Answer from the drawing. Dimensions are ordinates in mm from the lowest x, y and z of the part. A direction names the side the tool comes from. Round coordinates to 2 decimals unless told otherwise and drop trailing zeros. Order: outer loops, then holes, each group sorted by start corner. A loop starts at its lowest first (then second) coordinate and runs counter-clockwise, first axis right, second up. Notation, with made-up numbers: M -8,74.5 L -1,74.5 A15 cw -1,96.5 Z; hole C 32,4.25 d11. An arc over 180 degrees is marked long. Write item = value, one per line. Start each with the question number.
(1) A cutting plane is placed at C-C, the plane y = 20.5. Determine the outline of the cut face in (x, z).
(2) Each of these flat-tipped pins is pushed along its axis until it touches: pin 1 (1.5 mm diameter, centred on x = 3.5, y = 13, fed in from +Z); pin 2 (1.5 mm diameter, centred on x = 1.5, y = 11.5, fed in from -Z); pin 3 (2.5 mm diameter, centred on x = 2, z = 4.5, fed in from +Y). Where does it stop, or does it pass through?
(3) Which of the six approach directions +Z, -Z, +X, -X, +Y, -Y give full straight-line access (tool end or side, diameter ignored) to the marked faces 4, 5 and 6?
(4) Straight lines are drawn through the part: probe 1 along Y at (x, z) = (4.5, 0.3); probe 2 along Z at (x, y) = (4.4, 15.5); probe 3 along Z at (x, y) = (0.3, 20.5). For each, find the intervals that lie inside material, in ascending order. Write a range as from..to.
(5) A cutting plane is placed at B-B, the plane x = 1.25. Determine the outline of the cut face in (y, z), and give its area (3 significant figures).
(6) For a pull along Y with two mould halves and no side action, classify the marked faces 1, 2 and 3 as released by +Y, released by -Y, zero draft, split by the parting line, or undercut.
(7) A cutting plane is placed at A-A, the plane z = 0.8. Determine the outline of the cut face in (x, y).
(8) A cutting plane is placed at D-D, the plane z = 4.4. Determine the outline of the cut face in (x, y).
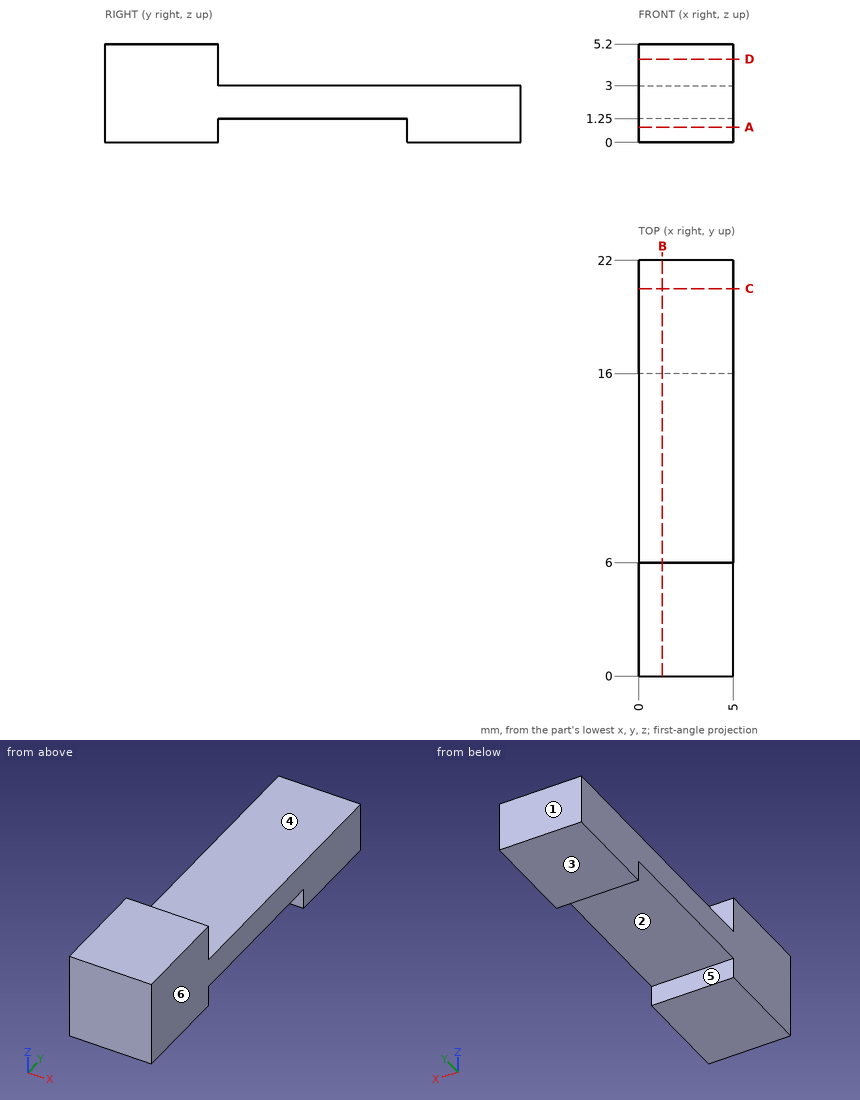
Reported:
q1.outline = M 0,0 L 5,0 L 5,3 L 0,3 Z
q2.pin_1 = 3
q2.pin_2 = 1.25
q2.pin_3 = 6
q3.face_4 = +Z, +X, -X, +Y
q3.face_5 = -Z, +X, -X
q3.face_6 = +Z, -Z, +X, +Y, -Y
q4.probe_1 = 0..6, 16..22
q4.probe_2 = 1.25..3
q4.probe_3 = 0..3
q5.outline = M 0,0 L 6,0 L 6,1.25 L 16,1.25 L 16,0 L 22,0 L 22,3 L 6,3 L 6,5.2 L 0,5.2 Z
q5.area = 66.7 mm²
q6.face_1 = released by +Y
q6.face_2 = undercut
q6.face_3 = zero draft
q7.outline = M 0,0 L 5,0 L 5,6 L 0,6 Z; M 0,16 L 5,16 L 5,22 L 0,22 Z
q8.outline = M 0,0 L 5,0 L 5,6 L 0,6 Z
